Work out the finished part from the listing and answer in its coordinate system (mm). Face numbers are marked on the shaded views. A direction names the side the tool comes from. Give positions to 0.01 mm unless a question says otherwise; leave off trailing zeros. Loops run counter-clockwise (first coordinate to the right, second up) from the corner with the lowest first, then second, coordinate; pieces in that order, holes last. Notation, with made-up numbers: M 63.25,45.5 L 88.25,45.5 A26 cw 88.25,68.5 Z; hole C 76,65.25 d11. An arc over 180 degrees is marked long. Answer in a Markdown table with one row per item. Add a question column.
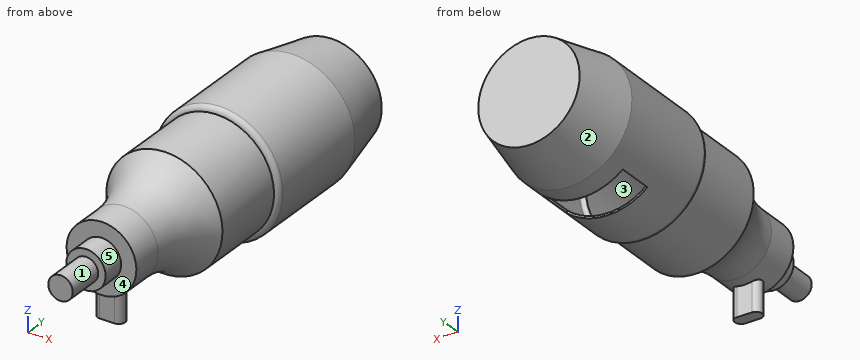
from build123d import *

# Parameters (mm, degrees)
ESQUISSE3_W             = 38
ESQUISSE3_H             = 17.5
ENL_V_MAT_EXTRU_1_DEPTH = 10
BOSS_EXTRU_1_REACH      = 188.017
BOSS_EXTRU_1_END_RADIUS = 16.5


with BuildPart() as part:
    # Esquisse1 → Révol.-Mince1 (revolve)
    with BuildSketch(Plane.XY, mode=Mode.PRIVATE) as r_vol_mince1_sk:
        with BuildLine():
            Line((0, 0), (0, -18))
            Line((0, -18), (5.8, -18))
            Line((5.8, -18), (5.8, 0))
            Line((5.8, 0), (9.3, 0))
            Line((9.3, 0), (9.3, 11))
            Line((9.3, 11), (16.5, 11))
            Line((16.5, 11), (16.5, 26.5))
            ThreePointArc((16.5, 26.5), (19.342380895, 42.008062419), (27.5, 55.5))
            Line((27.5, 55.5), (27.5, 92))
            ThreePointArc((27.5, 92), (29.267766953, 92.732233047), (30, 94.5))
            Line((30, 94.5), (30, 145.5))
            Line((30, 145.5), (24, 173.5))
            Line((24, 173.5), (0, 173.5))
            Line((0, 173.5), (0, 172.5))
            Line((0, 172.5), (23.19158421, 172.5))
            Line((23.19158421, 172.5), (29, 145.394059646))
            Line((29, 145.394059646), (29, 94.5))
            ThreePointArc((29, 94.5), (28.112372436, 93.130693606), (26.5, 93.381966011))
            Line((26.5, 93.381966011), (26.5, 55.876861643))
            ThreePointArc((26.5, 55.876861643), (18.340175363, 42.184387141), (15.5, 26.5))
            Line((15.5, 26.5), (15.5, 12))
            Line((15.5, 12), (8.3, 12))
            Line((8.3, 12), (8.3, 1))
            Line((8.3, 1), (4.8, 1))
            Line((4.8, 1), (4.8, -17))
            Line((4.8, -17), (1, -17))
            Line((1, -17), (1, 0))
            Line((1, 0), (0, 0))
        make_face()
    revolve(r_vol_mince1_sk.sketch.rotate(Axis((0, 182.175, 0), (0, -1, 0)), 90), axis=Axis((0, 182.175, 0), (0, -1, 0)))

    # Esquisse3 → Enlèv. mat.-Extru.1 (cut)
    with BuildSketch(Plane(origin=(0, 0, -30), x_dir=(-1, 0, 0), z_dir=(0, 0, -1))):
        with Locations((0, 126.75)):
            Rectangle(ESQUISSE3_W, ESQUISSE3_H)
    extrude(amount=-ENL_V_MAT_EXTRU_1_DEPTH, mode=Mode.SUBTRACT)

    # Boss.-Extru.1: up to this cylinder (the profile starts outside it)
    boss_extru_1_end = Plane(origin=(0, 18, 0), z_dir=(0, 1, 0)) * Cylinder(BOSS_EXTRU_1_END_RADIUS, 410.034, mode=Mode.PRIVATE)
    # Esquisse4 → Boss.-Extru.1 (add, up to the surface)
    with BuildSketch(Plane(origin=(0, 0, -30), x_dir=(-1, 0, 0), z_dir=(0, 0, -1)), mode=Mode.PRIVATE) as boss_extru_1_sk1:
        with BuildLine():
            Line((-3.5, 21), (3.5, 21))
            ThreePointArc((3.5, 21), (6.5, 18), (3.5, 15))
            Line((3.5, 15), (-3.5, 15))
            ThreePointArc((-3.5, 15), (-6.5, 18), (-3.5, 21))
        make_face()
    boss_extru_1_tool1 = extrude(boss_extru_1_sk1.sketch, amount=-BOSS_EXTRU_1_REACH, mode=Mode.PRIVATE) - boss_extru_1_end
    add(boss_extru_1_tool1.solids().sort_by_distance((0, 18, -30))[0])


solid = part.part
(1) The mould has two halves that part along Y. Classify the marked faces 3, 4 and 5: pulls with the +Y half, pulls with the -Y half, needs draft (parallel to the pull), parting line crosses it, or undercut.
(2) Each of these flat-tipped pins is pushed along its axis until it touches: P1, Ø5, axis at x = 7, z = 24, coming from the +Y side; P2, Ø6, axis at x = -16.5, y = 51, coming from the +Z side; P3, Ø5.5, axis at x = 0, z = -23.5, coming from the -Y side; P4, Ø1.5, axis at x = 8, y = 86.5, coming from the +Z side. Where does it stop, or does it pass through?
(3) Consider line 1 along X through (y, z) = (-4, 0); line 2 along X through (y, z) = (64.5, 0); line 3 along Y through (x, z) = (-12, 6). Determine where each line is inside the solid, lowest interval first. Write a range as from..to.
(4) Which of the six approach directions +Z, -Z, +X, -X, +Y, -Y give full straight-line access (tool end or side, diameter ignored) to the marked faces 1 and 2?
(5) Section A-A, the plane y = 18 is taken. Determine the outline of the cut face in (x, z), and give its area (3 significant figures).
Numbers:
| question | item | result |
|---|---|---|
| 1 | face 3 | undercut |
| 1 | face 4 | pulls with the -Y half |
| 1 | face 5 | needs draft |
| 2 | P1 | stops at y = 173.5 |
| 2 | P2 | stops at z = 21.15 |
| 2 | P3 | stops at y = 15 |
| 2 | P4 | stops at z = 26.53 |
| 3 | line 1 | x = -5.8..-4.8, -1..1, 4.8..5.8 |
| 3 | line 2 | x = -27.5..-26.5, 26.5..27.5 |
| 3 | line 3 | y = 11..12, 172.5..173.5 |
| 4 | face 1 | -Y |
| 4 | face 2 | +Y |
| 5 | outline | M -6.5,-30 L 6.5,-30 L 6.5,-15.17 A16.5 ccw long -6.5,-15.17 Z; hole C 0,0 d31 |
| 5 | area | 282 mm² |
